from build123d import *

# Parameters (mm, degrees)
ESTRUSIONE_ESTRUSIONE2_DEPTH = 450


with BuildPart() as part:
    # Schizzo1 → Estrusione-Estrusione2 (new body)
    with BuildSketch(Plane.XY):
        with BuildLine():
            Line((-15, 13), (-15, 4.7))
            Line((-15, 4.7), (-14.3, 4.7))
            Line((-14.3, 4.7), (-14.3, 4))
            Line((-14.3, 4), (-12.8, 4))
            Line((-12.8, 4), (-12.8, 8.25))
            Line((-12.8, 8.25), (-10.017766953, 8.25))
            Line((-10.017766953, 8.25), (-6, 4.232233047))
            Line((-6, 4.232233047), (-6, 1))
            Line((-6, 1), (-5, 0))
            Line((-5, 0), (-6, -1))
            Line((-6, -1), (-6, -4.232233047))
            Line((-6, -4.232233047), (-10.017766953, -8.25))
            Line((-10.017766953, -8.25), (-12.8, -8.25))
            Line((-12.8, -8.25), (-12.8, -4))
            Line((-12.8, -4), (-14.3, -4))
            Line((-14.3, -4), (-14.3, -4.7))
            Line((-14.3, -4.7), (-15, -4.7))
            Line((-15, -4.7), (-15, -13))
            ThreePointArc((-15, -13), (-14.414213562, -14.414213562), (-13, -15))
            Line((-13, -15), (-4.7, -15))
            Line((-4.7, -15), (-4.7, -14.3))
            Line((-4.7, -14.3), (-4, -14.3))
            Line((-4, -14.3), (-4, -12.8))
            Line((-4, -12.8), (-8.25, -12.8))
            Line((-8.25, -12.8), (-8.25, -10.017766953))
            Line((-8.25, -10.017766953), (-4.232233047, -6))
            Line((-4.232233047, -6), (-1, -6))
            Line((-1, -6), (0, -5))
            Line((0, -5), (1, -6))
            Line((1, -6), (4.232233047, -6))
            Line((4.232233047, -6), (8.25, -10.017766953))
            Line((8.25, -10.017766953), (8.25, -12.8))
            Line((8.25, -12.8), (4, -12.8))
            Line((4, -12.8), (4, -14.3))
            Line((4, -14.3), (4.7, -14.3))
            Line((4.7, -14.3), (4.7, -15))
            Line((4.7, -15), (13, -15))
            ThreePointArc((13, -15), (14.414213562, -14.414213562), (15, -13))
            Line((15, -13), (15, -4.7))
            Line((15, -4.7), (14.3, -4.7))
            Line((14.3, -4.7), (14.3, -4))
            Line((14.3, -4), (12.8, -4))
            Line((12.8, -4), (12.8, -8.25))
            Line((12.8, -8.25), (10.017766953, -8.25))
            Line((10.017766953, -8.25), (6, -4.232233047))
            Line((6, -4.232233047), (6, -1))
            Line((6, -1), (5, 0))
            Line((5, 0), (6, 1))
            Line((6, 1), (6, 4.232233047))
            Line((6, 4.232233047), (10.017766953, 8.25))
            Line((10.017766953, 8.25), (12.8, 8.25))
            Line((12.8, 8.25), (12.8, 4))
            Line((12.8, 4), (14.3, 4))
            Line((14.3, 4), (14.3, 4.7))
            Line((14.3, 4.7), (15, 4.7))
            Line((15, 4.7), (15, 13))
            ThreePointArc((15, 13), (14.414213562, 14.414213562), (13, 15))
            Line((13, 15), (4.7, 15))
            Line((4.7, 15), (4.7, 14.3))
            Line((4.7, 14.3), (4, 14.3))
            Line((4, 14.3), (4, 12.8))
            Line((4, 12.8), (8.25, 12.8))
            Line((8.25, 12.8), (8.25, 10.017766953))
            Line((8.25, 10.017766953), (4.232233047, 6))
            Line((4.232233047, 6), (1, 6))
            Line((1, 6), (0, 5))
            Line((0, 5), (-1, 6))
            Line((-1, 6), (-4.232233047, 6))
            Line((-4.232233047, 6), (-8.25, 10.017766953))
            Line((-8.25, 10.017766953), (-8.25, 12.8))
            Line((-8.25, 12.8), (-4, 12.8))
            Line((-4, 12.8), (-4, 14.3))
            Line((-4, 14.3), (-4.7, 14.3))
            Line((-4.7, 14.3), (-4.7, 15))
            Line((-4.7, 15), (-13, 15))
            ThreePointArc((-13, 15), (-14.414213562, 14.414213562), (-15, 13))
        make_face()
        with BuildLine():
            Line((13.5, 10.75), (13.5, 12.5))
            ThreePointArc((13.5, 12.5), (13.207106781, 13.207106781), (12.5, 13.5))
            Line((12.5, 13.5), (10.75, 13.5))
            ThreePointArc((10.75, 13.5), (10.042893219, 13.207106781), (9.75, 12.5))
            Line((9.75, 12.5), (9.75, 10.75))
            ThreePointArc((9.75, 10.75), (10.042893219, 10.042893219), (10.75, 9.75))
            Line((10.75, 9.75), (12.5, 9.75))
            ThreePointArc((12.5, 9.75), (13.207106781, 10.042893219), (13.5, 10.75))
        make_face(mode=Mode.SUBTRACT)
        with BuildLine():
            Line((10.75, -13.5), (12.5, -13.5))
            ThreePointArc((12.5, -13.5), (13.207106781, -13.207106781), (13.5, -12.5))
            Line((13.5, -12.5), (13.5, -10.75))
            ThreePointArc((13.5, -10.75), (13.207106781, -10.042893219), (12.5, -9.75))
            Line((12.5, -9.75), (10.75, -9.75))
            ThreePointArc((10.75, -9.75), (10.042893219, -10.042893219), (9.75, -10.75))
            Line((9.75, -10.75), (9.75, -12.5))
            ThreePointArc((9.75, -12.5), (10.042893219, -13.207106781), (10.75, -13.5))
        make_face(mode=Mode.SUBTRACT)
        with BuildLine():
            Line((-13.5, -10.75), (-13.5, -12.5))
            ThreePointArc((-13.5, -12.5), (-13.207106781, -13.207106781), (-12.5, -13.5))
            Line((-12.5, -13.5), (-10.75, -13.5))
            ThreePointArc((-10.75, -13.5), (-10.042893219, -13.207106781), (-9.75, -12.5))
            Line((-9.75, -12.5), (-9.75, -10.75))
            ThreePointArc((-9.75, -10.75), (-10.042893219, -10.042893219), (-10.75, -9.75))
            Line((-10.75, -9.75), (-12.5, -9.75))
            ThreePointArc((-12.5, -9.75), (-13.207106781, -10.042893219), (-13.5, -10.75))
        make_face(mode=Mode.SUBTRACT)
        with BuildLine():
            Line((1.995536102, 3.056196274), (3.00520382, 4.065863992))
            Line((3.00520382, 4.065863992), (4.065863992, 3.00520382))
            Line((4.065863992, 3.00520382), (3.056196274, 1.995536102))
            ThreePointArc((3.056196274, 1.995536102), (3.498400806, 1.041005187), (3.65, 0))
            ThreePointArc((3.65, 0), (3.498400806, -1.041005187), (3.056196274, -1.995536102))
            Line((3.056196274, -1.995536102), (4.065863992, -3.00520382))
            Line((4.065863992, -3.00520382), (3.00520382, -4.065863992))
            Line((3.00520382, -4.065863992), (1.995536102, -3.056196274))
            ThreePointArc((1.995536102, -3.056196274), (1.041005187, -3.498400806), (0, -3.65))
            ThreePointArc((0, -3.65), (-1.041005187, -3.498400806), (-1.995536102, -3.056196274))
            Line((-1.995536102, -3.056196274), (-3.00520382, -4.065863992))
            Line((-3.00520382, -4.065863992), (-4.065863992, -3.00520382))
            Line((-4.065863992, -3.00520382), (-3.056196274, -1.995536102))
            ThreePointArc((-3.056196274, -1.995536102), (-3.498400806, -1.041005187), (-3.65, 0))
            ThreePointArc((-3.65, 0), (-3.498400806, 1.041005187), (-3.056196274, 1.995536102))
            Line((-3.056196274, 1.995536102), (-4.065863992, 3.00520382))
            Line((-4.065863992, 3.00520382), (-3.00520382, 4.065863992))
            Line((-3.00520382, 4.065863992), (-1.995536102, 3.056196274))
            ThreePointArc((-1.995536102, 3.056196274), (-1.041005187, 3.498400806), (0, 3.65))
            ThreePointArc((0, 3.65), (1.041005187, 3.498400806), (1.995536102, 3.056196274))
        make_face(mode=Mode.SUBTRACT)
        with BuildLine():
            Line((-10.75, 9.75), (-12.5, 9.75))
            ThreePointArc((-12.5, 9.75), (-13.207106781, 10.042893219), (-13.5, 10.75))
            Line((-13.5, 10.75), (-13.5, 12.5))
            ThreePointArc((-13.5, 12.5), (-13.207106781, 13.207106781), (-12.5, 13.5))
            Line((-12.5, 13.5), (-10.75, 13.5))
            ThreePointArc((-10.75, 13.5), (-10.042893219, 13.207106781), (-9.75, 12.5))
            Line((-9.75, 12.5), (-9.75, 10.75))
            ThreePointArc((-9.75, 10.75), (-10.042893219, 10.042893219), (-10.75, 9.75))
        make_face(mode=Mode.SUBTRACT)
    extrude(amount=ESTRUSIONE_ESTRUSIONE2_DEPTH)


solid = part.part
Verification items for the finished model (mm, model axes). Coordinates: 2 decimals unless noted, no trailing zeros. Answer as a JSON object with one key per item and string values. Group by question number.
Item 1: Depth check by flat-ended pin: pin 1 (12 mm diameter, centred on y = -3, z = 91.5, fed in from -X); pin 2 (0.8 mm diameter, centred on y = -13.5, z = 244.5, fed in from +X); pin 3 (1.6 mm diameter, centred on x = -3, z = 221.5, fed in from -Y); pin 4 (0.8 mm diameter, centred on y = 4, z = 190.5, fed in from +X). Enter the tip coordinate at first touch or a pass-through.
Item 2: Sectioned sample at A-A on z = 362. State how many separate pieces and enclosed holes the cut face has, plus the area to 3 significant figures.
Item 3: Scan lines: probe 1 along Y at (x, z) = (-6.5, 54); probe 2 along X at (y, z) = (12.5, 376). Record each from-to range of solid material in increasing order.
Evaluation:
{
 "1": {"pin 1": "stops at x = -15", "pin 2": "stops at x = 15", "pin 3": "stops at y = -6", "pin 4": "stops at x = 14.3"},
 "2": {"separate pieces": "1", "enclosed holes": "5", "area": "331 mm²"},
 "3": {"probe 1": "y = -15 to -12.8, -8.27 to -4.73, 4.73 to 8.27, 12.8 to 15", "probe 2": "x = -15 to -13.5, -9.75 to -8.25, 8.25 to 9.75, 13.5 to 15"}
}
